The listing builds one solid part. Answer for the finished solid, in the listing's coordinates (mm). Round coordinates to 2 decimals unless told otherwise and drop trailing zeros. Write each loop counter-clockwise with the first axis right and the second up, starting at its lowest first coordinate (ties: lowest second). Pieces come first, ordered by that corner, then holes. Notation, with made-up numbers: (56, 3) - (90, 3) arc R13 cw to (90, 15) - close; hole circle Ø3 at (-7, 64). An arc over 180 degrees is marked (long way). Answer as CSV lines item,"result". Start each with the question number.
Item 1: A cutting plane is placed at A-A on x = 57.7. Determine the outline of the cut face in (y, z).
Item 2: A cutting plane is placed at B-B on y = 12.7. Determine the outline of the cut face in (x, z) (3 decimals).
Item 3: Straight lines are drawn through the part: line 1 along X through (y, z) = (13.5, -0.5); line 2 along Y through (x, z) = (103, -2.75); line 3 along Y through (x, z) = (57.7, -4.25). For each, find the intervals that lie inside material, in ascending order. Write a range as [from, to].
Item 4: A cutting plane is placed at C-C on z = -2. Determine the outline of the cut face in (x, y) (3 decimals), and give its area (3 significant figures).
Item 5: For a pull along X with two mould halves and no side action, classify faces 1 (the flat face through (0, 13, -3)), 2 (the cylindrical face through (10.18, 10.77, -3.13)), 3 (the cylindrical face through (34.589, 11.787, -3.131)), 4 (the flat face through (57, 18, 0)) as pulls with the +X half, pulls with the -X half, needs draft (parallel to the pull), parting line crosses it, or undercut.
Item 6: A cutting plane is placed at D-D on x = 102.7. Determine the outline of the cut face in (y, z) (3 decimals), and give its area (3 significant figures).
```python
from build123d import *

# Parameters (mm, degrees)
SKETCH1_W           = 6.35
SKETCH1_H           = 25.4
BOSS_EXTRUDE1_DEPTH = 115.4
SKETCH2_R           = 5
SKETCH2_R_2         = 1.5
SKETCH2_R_3         = 3.175
CUT_EXTRUDE1_DEPTH  = 119.332761736


with BuildPart() as part:
    # Sketch1 → Boss-Extrude1 (new body)
    with BuildSketch(Plane(origin=(0, 0, 0), x_dir=(0, 0, -1), z_dir=(1, 0, 0))):
        with Locations((3.175, 12.7)):
            Rectangle(SKETCH1_W, SKETCH1_H)
    extrude(amount=BOSS_EXTRUDE1_DEPTH)

    # Sketch2 → Cut-Extrude1 (cut, through all)
    with BuildSketch(Plane.XY):
        with Locations((57.7, 12.7)):
            Circle(SKETCH2_R)
        with Locations((35.779689783, 12.7)):
            Circle(SKETCH2_R_2)
        with Locations((12.7, 12.7)):
            Circle(SKETCH2_R_3)
        with Locations((79.620310217, 12.7)):
            Circle(SKETCH2_R_2)
        with Locations((102.7, 12.7)):
            Circle(SKETCH2_R_3)
    extrude(amount=-CUT_EXTRUDE1_DEPTH, mode=Mode.SUBTRACT)


solid = part.part
```
Geometry says:
1,outline,"(0, -6.35) - (7.7, -6.35) - (7.7, 0) - (0, 0) - close; (17.7, -6.35) - (25.4, -6.35) - (25.4, 0) - (17.7, 0) - close"
2,outline,"(0, -6.35) - (9.525, -6.35) - (9.525, 0) - (0, 0) - close; (15.875, -6.35) - (34.28, -6.35) - (34.28, 0) - (15.875, 0) - close; (37.28, -6.35) - (52.7, -6.35) - (52.7, 0) - (37.28, 0) - close; (62.7, -6.35) - (78.12, -6.35) - (78.12, 0) - (62.7, 0) - close; (81.12, -6.35) - (99.525, -6.35) - (99.525, 0) - (81.12, 0) - close; (105.875, -6.35) - (115.4, -6.35) - (115.4, 0) - (105.875, 0) - close"
3,line 1,"x = [0, 9.63], [15.77, 34.51], [37.05, 52.76], [62.64, 78.35], [80.89, 99.63], [105.77, 115.4]"
3,line 2,"y = [0, 9.54], [15.86, 25.4]"
3,line 3,"y = [0, 7.7], [17.7, 25.4]"
4,outline,"(0, 0) - (115.4, 0) - (115.4, 25.4) - (0, 25.4) - close; hole circle Ø6.35 at (12.7, 12.7); hole circle Ø3 at (35.78, 12.7); hole circle Ø10 at (57.7, 12.7); hole circle Ø3 at (79.62, 12.7); hole circle Ø6.35 at (102.7, 12.7)"
4,area,"2,780 mm^2"
5,face 1,"pulls with the -X half"
5,face 2,"undercut"
5,face 3,"undercut"
5,face 4,"needs draft"
6,outline,"(0, -6.35) - (9.525, -6.35) - (9.525, 0) - (0, 0) - close; (15.875, -6.35) - (25.4, -6.35) - (25.4, 0) - (15.875, 0) - close"
6,area,"121 mm^2"
